Input: dimensioned drawing with shaded views. Units: mm. Origin: part minimum x, y, z. Round coordinates to 2 decimals unless told otherwise and drop trailing zeros. Write each loop counter-clockwise with the first axis right and the second up, starting at its lowest first coordinate (ties: lowest second). Pieces come first, ordered by that corner, then holes. Notation, with made-up numbers: (52, -3) -> (95, -3) arc R15 cw to (95, 26) -> close; hole circle Ø2 at (48.25, -1.5). An arc over 180 degrees is marked (long way). Return JSON: item names as keys, results as strings. Group by question number.
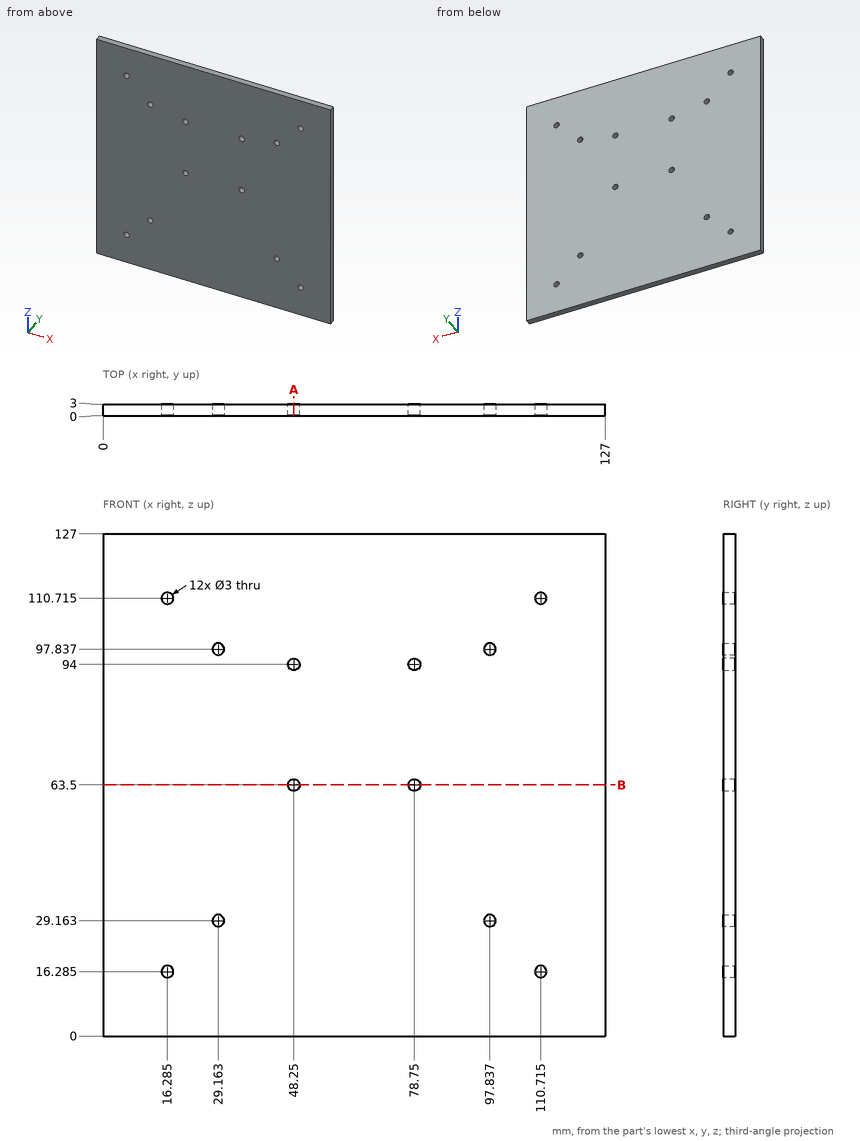
Item 1: Cut plane B-B on z = 63.5. Output: boundary loops of the cut face in (x, y), and give its area (3 significant figures).
Item 2: Material intervals for probe 1 along X at (y, z) = (1.85, 63.5); probe 2 along Z at (x, y) = (78.75, 2.1), sorted ascending.
Item 3: Cut plane A-A on x = 48.25. Output: boundary loops of the cut face in (y, z), and give its area (3 significant figures).
Item 4: First-contact query: pin 1 Ø1 at (y, z) = (1.5, 89.5) entering from -X. Flat tip, straight axial feed; report the tip coordinate or a pass-through.
Here are the results:
{
 "1": {"outline": "(0, 0) -> (46.75, 0) -> (46.75, 3) -> (0, 3) -> close; (49.75, 0) -> (77.25, 0) -> (77.25, 3) -> (49.75, 3) -> close; (80.25, 0) -> (127, 0) -> (127, 3) -> (80.25, 3) -> close", "area": "363 mm^2"},
 "2": {"probe 1": "x = 0 to 46.75, 49.75 to 77.25, 80.25 to 127", "probe 2": "z = 0 to 62, 65 to 92.5, 95.5 to 127"},
 "3": {"outline": "(0, 0) -> (3, 0) -> (3, 62) -> (0, 62) -> close; (0, 65) -> (3, 65) -> (3, 92.5) -> (0, 92.5) -> close; (0, 95.5) -> (3, 95.5) -> (3, 127) -> (0, 127) -> close", "area": "363 mm^2"},
 "4": {"pin 1": "stops at x = 0"}
}
